Can you work these out from the model? Positions are in its coordinate system, mm. Round coordinates to 2 decimals unless told otherwise and drop trailing zeros. Write each loop counter-clockwise with the first axis right and the second up, starting at its lowest first coordinate (ties: lowest second). Pieces come first, ordered by that corner, then holes. Notation, with made-up numbers: M -35.5,66.5 L -12.5,66.5 A23 ccw -12.5,79.5 Z; hole C 40.25,30.25 d2. An arc over 180 degrees is marked long. Use one line per item in the form item = value. Start each with the question number.
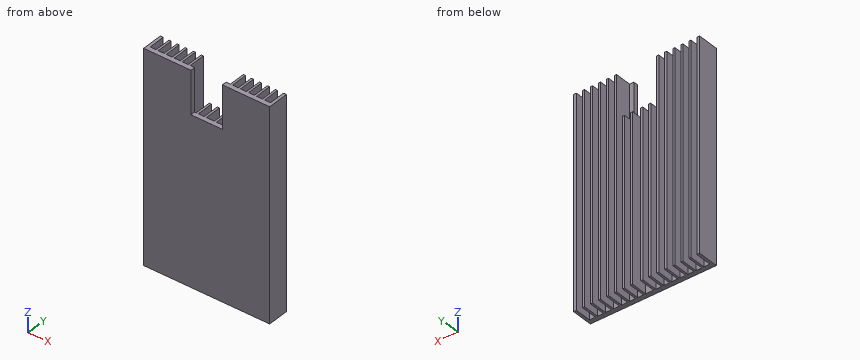
Autodesk Inventor part; units mm, degrees
ref_plane "YZ Plane" through (0, 0, 0) normal (1, 0, 0) x (0, 1, 0)
ref_plane "XZ Plane" through (0, 0, 0) normal (0, 1, 0) x (-1, 0, 0)
ref_plane "XY Plane" through (0, 0, 0) normal (0, 0, 1) x (1, 0, 0)
sketch "Sketch1" plane through (0, 0, 0) normal (0, 1, 0) x (-1, 0, 0)
  line L0 (0, 0) -> (60, 0)
  line L1 (60, 0) -> (60, -100)
  line L2 (60, -100) -> (0, -100)
  line L3 (0, -100) -> (0, 0)
  dimension "d0" = 60
  dimension "d1" = 100
extrude "Extrusion1" add sketch "Sketch1" along normal blind 10
sketch "Sketch2" plane through (0, 10, 0) normal (0, 1, 0) x (1, 0, 0)
  line L0 (-60, 0) -> (0, 0)
  line L1 (-30, 0) -> (-30, 100)
  line L2 (0, 100) -> (-60, 100)
  line L3 (-31.9, 0) -> (-28.1, 0)
  line L4 (-28.1, 0) -> (-28.1, 100)
  line L5 (-28.1, 100) -> (-31.9, 100)
  line L6 (-31.9, 100) -> (-31.9, 0)
  line L7 (-31.9, 0) -> (-28.1, 100) construction
  line L8 (-28.1, 0) -> (-31.9, 100) construction
  line L9 (-32.9, 0) -> (-35.72, 0)
  line L10 (-35.72, 0) -> (-35.72, 100)
  line L11 (-35.72, 100) -> (-32.9, 100)
  line L12 (-32.9, 100) -> (-32.9, 0)
  line L13 (-32.9, 0) -> (-35.72, 100) construction
  line L14 (-35.72, 0) -> (-32.9, 100) construction
  line L15 (-39.54, 0) -> (-36.72, 0)
  line L16 (-36.72, 0) -> (-36.72, 100)
  line L17 (-36.72, 100) -> (-39.54, 100)
  line L18 (-39.54, 100) -> (-39.54, 0)
  line L19 (-39.54, 0) -> (-36.72, 100) construction
  line L20 (-36.72, 0) -> (-39.54, 100) construction
  line L21 (-43.36, 0) -> (-40.54, 0)
  line L22 (-40.54, 0) -> (-40.54, 100)
  line L23 (-40.54, 100) -> (-43.36, 100)
  line L24 (-43.36, 100) -> (-43.36, 0)
  line L25 (-43.36, 0) -> (-40.54, 100) construction
  line L26 (-40.54, 0) -> (-43.36, 100) construction
  line L27 (-47.18, 0) -> (-44.36, 0)
  line L28 (-44.36, 0) -> (-44.36, 100)
  line L29 (-44.36, 100) -> (-47.18, 100)
  line L30 (-47.18, 100) -> (-47.18, 0)
  line L31 (-47.18, 0) -> (-44.36, 100) construction
  line L32 (-44.36, 0) -> (-47.18, 100) construction
  line L33 (-51, 0) -> (-48.18, 0)
  line L34 (-48.18, 0) -> (-48.18, 100)
  line L35 (-48.18, 100) -> (-51, 100)
  line L36 (-51, 100) -> (-51, 0)
  line L37 (-51, 0) -> (-48.18, 100) construction
  line L38 (-48.18, 0) -> (-51, 100) construction
  line L39 (-54.82, 0) -> (-52, 0)
  line L40 (-52, 0) -> (-52, 100)
  line L41 (-52, 100) -> (-54.82, 100)
  line L42 (-54.82, 100) -> (-54.82, 0)
  line L43 (-54.82, 0) -> (-52, 100) construction
  line L44 (-52, 0) -> (-54.82, 100) construction
  line L45 (-58.64, 0) -> (-55.82, 0)
  line L46 (-55.82, 0) -> (-55.82, 100)
  line L47 (-55.82, 100) -> (-58.64, 100)
  line L48 (-58.64, 100) -> (-58.64, 0)
  line L49 (-58.64, 0) -> (-55.82, 100) construction
  line L50 (-55.82, 0) -> (-58.64, 100) construction
  line L51 (-31.9, 0) -> (-31.9, 100)
  line L52 (-28.1, 100) -> (-28.1, 0)
  line L53 (-28.1, 0) -> (-31.9, 100) construction
  line L54 (-31.9, 0) -> (-28.1, 100) construction
  line L55 (-24.28, 0) -> (-24.28, 100)
  line L56 (-27.1, 100) -> (-27.1, 0)
  line L57 (-27.1, 0) -> (-24.28, 100) construction
  line L58 (-24.28, 0) -> (-27.1, 100) construction
  line L59 (-23.28, 0) -> (-23.28, 100)
  line L60 (-20.46, 100) -> (-20.46, 0)
  line L61 (-20.46, 0) -> (-23.28, 100) construction
  line L62 (-23.28, 0) -> (-20.46, 100) construction
  line L63 (-19.46, 0) -> (-19.46, 100)
  line L64 (-16.64, 100) -> (-16.64, 0)
  line L65 (-16.64, 0) -> (-19.46, 100) construction
  line L66 (-19.46, 0) -> (-16.64, 100) construction
  line L67 (-15.64, 0) -> (-15.64, 100)
  line L68 (-12.82, 100) -> (-12.82, 0)
  line L69 (-12.82, 0) -> (-15.64, 100) construction
  line L70 (-15.64, 0) -> (-12.82, 100) construction
  line L71 (-11.82, 0) -> (-11.82, 100)
  line L72 (-9, 100) -> (-9, 0)
  line L73 (-9, 0) -> (-11.82, 100) construction
  line L74 (-11.82, 0) -> (-9, 100) construction
  line L75 (-8, 0) -> (-8, 100)
  line L76 (-5.18, 100) -> (-5.18, 0)
  line L77 (-5.18, 0) -> (-8, 100) construction
  line L78 (-8, 0) -> (-5.18, 100) construction
  line L79 (-4.18, 0) -> (-4.18, 100)
  line L80 (-1.36, 100) -> (-1.36, 0)
  line L81 (-1.36, 0) -> (-4.18, 100) construction
  line L82 (-4.18, 0) -> (-1.36, 100) construction
  line L83 (-60, 100) -> (-60, 0)
  point P0 (-30, 50)
  point P1 (-34.31, 50)
  point P2 (-38.13, 50)
  point P3 (-41.95, 50)
  point P4 (-45.77, 50)
  point P5 (-49.59, 50)
  point P6 (-53.41, 50)
  point P7 (-57.23, 50)
  point P8 (-25.69, 50)
  point P9 (-21.87, 50)
  point P10 (-18.05, 50)
  point P11 (-14.23, 50)
  point P12 (-10.41, 50)
  point P13 (-6.59, 50)
  point P14 (-2.77, 50)
  point P15 (-1.36, 0)
  point P16 (-1.36, 100)
  point P17 (-4.18, 100)
  point P18 (-4.18, 0)
  point P19 (-5.18, 0)
  point P20 (-5.18, 100)
  point P21 (-8, 100)
  point P22 (-8, 0)
  point P23 (-9, 0)
  point P24 (-9, 100)
  point P25 (-11.82, 100)
  point P26 (-11.82, 0)
  point P27 (-12.82, 0)
  point P28 (-12.82, 100)
  point P29 (-15.64, 100)
  point P30 (-15.64, 0)
  point P31 (-16.64, 0)
  point P32 (-16.64, 100)
  point P33 (-19.46, 100)
  point P34 (-19.46, 0)
  point P35 (-23.28, 0)
  point P36 (-20.46, 0)
  point P37 (-27.1, 0)
  point P38 (-24.28, 0)
  point P39 (-31.9, 0)
  point P40 (-28.1, 0)
  point P41 (-32.9, 0)
  point P42 (-35.72, 0)
  point P43 (-39.54, 0)
  point P44 (-36.72, 0)
  point P45 (-43.36, 0)
  point P46 (-40.54, 0)
  point P47 (-47.18, 0)
  point P48 (-44.36, 0)
  point P49 (-51, 0)
  point P50 (-48.18, 0)
  point P51 (-54.82, 100)
  point P52 (-54.82, 0)
  point P53 (-52, 0)
  point P54 (-52, 100)
  point P55 (-58.64, 100)
  point P56 (-58.64, 0)
  point P57 (-55.82, 0)
  point P58 (-55.82, 100)
  dimension "d4" = 3.8
  dimension "d5" = 100
  dimension "d6" = 2.82
  dimension "d7" = 1
  dimension "d8" = 100
  dimension "d9" = 2.82
  dimension "d10" = 1
  dimension "d11" = 2.82
  dimension "d12" = 1
  dimension "d13" = 2.82
  dimension "d14" = 100
  dimension "d15" = 1
  dimension "d16" = 2.82
  dimension "d17" = 100
  dimension "d18" = 1
  dimension "d19" = 2.82
  dimension "d20" = 100
  dimension "d21" = 1
  dimension "d22" = 2.82
  dimension "d23" = 100
  dimension "d24" = 1
  dimension "d27" = 1.36
  dimension "d28" = 0
  dimension "d29" = 0
  dimension "d30" = 100
  dimension "d31" = 100
extrude "Extrusion2" cut sketch "Sketch2" against normal blind 7.8 contours L48 L2 L46 L0 | L42 L2 L40 L0 | L36 L2 L34 L0 | L30 L2 L28 L0 | L24 L2 L22 L0 | L18 L2 L16 L0 | L10 L2 L12 L0 | L6 L2 L1 L0 | L1 L2 L4 L0 | L56 L2 L55 L0 | L59 L2 L60 L0 | L63 L2 L64 L0 | L67 L2 L68 L0 | L71 L2 L72 L0 | L75 L2 L76 L0 | L79 L2 L80 L0
sketch "Sketch3" plane through (0, 0, 0) normal (0, -1, 0) x (1, 0, 0)
  line L0 (-12.82, 0) -> (-11.82, 0)
  line L1 (-22.5, 0) -> (-37.5, 0)
  line L2 (-37.5, 0) -> (-37.5, -15.5)
  line L3 (-37.5, -15.5) -> (-22.5, -15.5)
  line L4 (-22.5, -15.5) -> (-22.5, 0)
  line L5 (0, 0) -> (0, -100)
  dimension "d32" = 15
  dimension "d33" = 15.5
  dimension "d34" = 22.5
extrude "Extrusion3" cut sketch "Sketch3" against normal blind 31.5
sketch "Sketch4" plane through (-37.5, 0, -15.5) normal (0, 0, 1) x (1, 0, 0)
  line L0 (0, -3.5749) -> (15, -3.5749)
  line L1 (15, -3.5749) -> (15, 11.2742)
  line L2 (15, 11.2742) -> (0, 11.2742)
  line L3 (0, 11.2742) -> (0, -3.5749)
  line L4 (0, 0) -> (0, 2.2)
  line L5 (15, 0) -> (15, 2.2)
  point P0 (37.5, 0)
  dimension "d37" = 0
  dimension "d38" = 0
extrude "Extrusion4" cut sketch "Sketch4" against normal blind 5
properties part number "heatsink" material "Aluminum 6061"
1. If we section it at A-A (y = 3.5): State how many separate pieces and enclosed holes the cut face has, and give its area (3 significant figures).
2. Please list where this line runs through material, in increasing order: line 1 along Y through (x, z) = (-45, -94.5).
3. Will this pin go through, and if not, where does the flat tip stop? pin 1 (2.5 mm diameter, centred on x = -38, z = -31.5, fed in from +Y).
4. If we section it at B-B (x = -7): List the corners of the cut face in (y, z) for me.
Model answer:
q1.separate_pieces = 16
q1.enclosed_holes = 0
q1.area = 1,590 mm2
q2.line_1 = 0 to 2.2
q3.pin_1 = 2.2
q4.outline = M 0,-100 L 2.2,-100 L 2.2,0 L 0,0 Z
